```python
from build123d import *

# Parameters (mm, degrees)
BOSS_EXTRUDE1_DEPTH = 5.842


with BuildPart() as part:
    # Sketch1 → Boss-Extrude1 (new body)
    with BuildSketch(Plane(origin=(0, 0, 0), x_dir=(1, 0, 0), z_dir=(0, 1, 0))):
        with BuildLine():
            Line((-2.4765, -2.032), (2.4765, -2.032))
            Line((2.4765, -2.032), (2.560704247, -2.032))
            ThreePointArc((2.560704247, -2.032), (3.26898, 0), (2.560704247, 2.032))
            Line((2.560704247, 2.032), (2.419800194, 2.032))
            Line((2.419800194, 2.032), (-2.533199806, 2.032))
            Line((-2.533199806, 2.032), (-2.560704247, 2.032))
            ThreePointArc((-2.560704247, 2.032), (-3.26898, 0), (-2.560704247, -2.032))
            Line((-2.560704247, -2.032), (-2.4765, -2.032))
        make_face()
        with BuildLine():
            Line((1.999998, -1.4605), (-1.999998, -1.4605))
            ThreePointArc((-1.999998, -1.4605), (-2.4765, 0), (-1.999998, 1.4605))
            Line((-1.999998, 1.4605), (1.999998, 1.4605))
            ThreePointArc((1.999998, 1.4605), (2.4765, 0), (1.999998, -1.4605))
        make_face(mode=Mode.SUBTRACT)
    extrude(amount=BOSS_EXTRUDE1_DEPTH)


solid = part.part
```
Can you work these out from the model? Positions are in its coordinate system, mm. A direction names the side the tool comes from. Round coordinates to 2 decimals unless told otherwise and drop trailing zeros. Loops run counter-clockwise (first coordinate to the right, second up) from the corner with the lowest first, then second, coordinate; pieces in that order, holes last.
Item 1: Please list where these lines run through material, in increasing order: L1, parallel to Z at x = 0.5, y = 4.4; L2, parallel to X at y = 3.95, z = 0.45; L3, parallel to X at y = 1.8, z = -1.2.
Item 2: Suppose I cut it at C-C, the plane z = 0.9. Write out the boundary of the cut face in (x, y).
Item 3: Suppose I cut it at D-D, the plane z = -1.75. Write out the boundary of the cut face in (x, y), then the cut area to 3 significant figures.
Item 4: Suppose I cut it at B-B, the plane y = 3.05. Write out the boundary of the cut face in (x, z).
Item 5: Which directions (+Z, -Z, +X, -X, +Y, -Y) give clear straight access to the entire face, cutting with the end or side of a thin tool? Please do faces 4 (the cylindrical face through (2.476, 2.88, -0.022)), 5 (the flat face through (0, 0, 1.8)).
Item 6: If we mould it in two halves opening along X, with no side actions, what happens to faces 1 (the flat face through (0, 3, -2.032)), 2 (the cylindrical face through (-2.476, 2.88, 0.022)), 3 (the cylindrical face through (3.27, 2.88, 0.03))? For each: +X half, -X half, draft (parallel to the pull), parting line (faces both ways), or undercut.
Item 7: Suppose I cut it at A-A, the plane x = 1.5. Write out the boundary of the cut face in (y, z), then the cut area to 3 significant figures.
Reported:
1. L1: z = -2.03 to -1.46, 1.46 to 2.03
1. L2: x = -3.24 to -2.44, 2.44 to 3.24
1. L3: x = -3.04 to -2.17, 2.17 to 3.04
2. outline: (-3.14, 0) - (-2.31, 0) - (-2.31, 5.84) - (-3.14, 5.84) - close; (2.31, 0) - (3.14, 0) - (3.14, 5.84) - (2.31, 5.84) - close
3. outline: (-2.76, 0) - (2.76, 0) - (2.76, 5.84) - (-2.76, 5.84) - close
3. area: 32.3 mm2
4. outline: (-2.56, -2.03) - (2.56, -2.03) arc R3.27 ccw to (2.56, 2.03) - (-2.56, 2.03) arc R3.27 ccw to start; hole (-2, -1.46) - (2, -1.46) arc R2.48 ccw to (2, 1.46) - (-2, 1.46) arc R2.48 ccw to start
5. face 4: +Y, -Y
5. face 5: +Z, -Z, +X, -X, -Y
6. face 1: draft
6. face 2: undercut
6. face 3: +X half
7. outline: (0, -2.03) - (5.84, -2.03) - (5.84, -1.46) - (0, -1.46) - close; (0, 1.46) - (5.84, 1.46) - (5.84, 2.03) - (0, 2.03) - close
7. area: 6.68 mm2
